```python
from build123d import *

# Parameters (mm, degrees)
F0_R     = 41.5
F0_R_2   = 26.5
F1_DEPTH = 2.5
F0_R_3   = 24.35
F2_DEPTH = 15
F3_R     = 2.49999
F4_R     = 2


# Not quite as in the source:
# - a fillet or chamfer is up to 0.001 mm smaller than in the source, because OpenCascade refuses the exact size


with BuildPart() as f1:
    # F0 (on Top) → F1 (new body)
    with BuildSketch(Plane.XY):
        Circle(F0_R)
        Circle(F0_R_2, mode=Mode.SUBTRACT)
    extrude(amount=F1_DEPTH)

    # F0 (on Top) → F2 (join)
    with BuildSketch(Plane.XY):
        Circle(F0_R_2)
        Circle(F0_R_3, mode=Mode.SUBTRACT)
    extrude(amount=F2_DEPTH)

    # F3 (radius 2.5 in the source; OpenCascade refuses exactly that, so slightly less here)
    f3_edges = [f1.edges().sort_by_distance(p)[0] for p in [
        (-41.5, 0, 0),
    ]]
    fillet(f3_edges, radius=F3_R)

    # F4
    f4_edges = [f1.edges().sort_by_distance(p)[0] for p in [
        (-24.35, 0, 15),
    ]]
    fillet(f4_edges, radius=F4_R)


solid = f1.part
```
Here's how the part is built. I have some questions about the finished solid (model axes, mm). Round coordinates to 2 decimals unless told otherwise and drop trailing zeros. Write each loop counter-clockwise with the first axis right and the second up, starting at its lowest first coordinate (ties: lowest second). Pieces come first, ordered by that corner, then holes.
Q1. If we mould it in two halves opening along Y, with no side actions, what happens to faces 1 (the cylindrical face through (14.246, 22.345, 8.662)), 2 (the flat face through (-18, -17, 0)), 3 (the cylindrical face through (-19.32, -14.82, 6.41))? For each: +Y half, -Y half, draft (parallel to the pull), parting line (faces both ways), or undercut.
Q2. If we section it at C-C on z = 3.5: Write out the boundary of the cut face in (x, y), plus the area to 3 significant figures.
Q3. Will these pins go through, and if not, where does the flat tip stop? P1, Ø1, axis at y = 12, z = 12, coming from the +X side; P2, Ø6, axis at x = 4.5, z = 11, coming from the -Y side; P3, Ø5, axis at x = 19, z = 8, coming from the -Y side.
Q4. Please list where these lines run through material, in increasing order: probe 1 along Y at (x, z) = (0, 6.75); probe 2 along Z at (x, y) = (-27.5, -16); probe 3 along X at (y, z) = (-15.5, 1.25).
Answer below:
1. face 1: parting line
1. face 2: draft
1. face 3: undercut
2. outline: circle Ø53 at (0, 0); hole circle Ø48.7 at (0, 0)
2. area: 343 mm2
3. P1: stops at x = 23.87
3. P2: stops at y = -26.46
3. P3: stops at y = -20.74
4. probe 1: y = -26.5 to -24.35, 24.35 to 26.5
4. probe 2: z = 0 to 2.5
4. probe 3: x = -38.14 to -18.78, 18.78 to 38.14
